Read the model definition and answer for the solid it produces. Units are mm, in the model's axes. Coordinates: 2 decimals unless noted, no trailing zeros. Write each loop counter-clockwise with the first axis right and the second up, starting at its lowest first coordinate (ties: lowest second). Pieces come first, ordered by that corner, then holes. Notation, with made-up numbers: (20, 16.25) -> (56, 16.25) arc R32 ccw to (56, 49.25) -> close; hole circle Ø7 at (28.5, -13). An arc over 180 degrees is marked (long way). Use CSV: the item, a comma, the result in double quotes.
from build123d import *

# Parameters (mm, degrees)
SKETCH1_R           = 100
BOSS_EXTRUDE1_DEPTH = 10
SKETCH2_R           = 15
CUT_EXTRUDE1_DEPTH  = 142.774468788
SKETCH3_R           = 10
CUT_EXTRUDE2_DEPTH  = 7.342697
CIRPATTERN1_START   = 2.65730266
CIRPATTERN1_DEPTH   = 7.34269734


# Read off the part's stored shape, not the designer's step: CirPattern1
with BuildPart() as part:
    # Sketch1 → Boss-Extrude1 (new body)
    with BuildSketch(Plane(origin=(0, 0, 0), x_dir=(1, 0, 0), z_dir=(0, 1, 0))):
        with Locations(Location((0, 0, 0), (0, 0, 270))):
            Circle(SKETCH1_R)
    extrude(amount=BOSS_EXTRUDE1_DEPTH)

    # Sketch2 → Cut-Extrude1 (cut, through all)
    with BuildSketch(Plane(origin=(0, 0, 0), x_dir=(1, 0, 0), z_dir=(0, 1, 0))):
        with Locations(Location((0, 0, 0), (0, 0, 270))):
            Circle(SKETCH2_R)
    extrude(amount=CUT_EXTRUDE1_DEPTH, mode=Mode.SUBTRACT)

    # Sketch3 → Cut-Extrude2 (cut)
    with BuildSketch(Plane(origin=(0, 10, 0), x_dir=(1, 0, 0), z_dir=(0, 1, 0))):
        with Locations((-21.793050468, 0)):
            Circle(SKETCH3_R)
    extrude(amount=-CUT_EXTRUDE2_DEPTH, mode=Mode.SUBTRACT)

    # CirPattern1 outline → CirPattern1 (cut)
    with BuildSketch(Plane(origin=(0, 0, 0), x_dir=(1, 0, 0), z_dir=(0, 1, 0)).offset(CIRPATTERN1_START)):
        with BuildLine():
            ThreePointArc((-13.764411953, -5.961624242), (-18.175613412, -9.322775829), (-23.699395197, -9.816610911))
            ThreePointArc((-23.699395197, -9.816610911), (-22.48108158, -22.48108158), (-9.816610911, -23.699395197))
            ThreePointArc((-9.816610911, -23.699395197), (0, -31.793050468), (9.816610911, -23.699395197))
            ThreePointArc((9.816610911, -23.699395197), (22.48108158, -22.48108158), (23.699395197, -9.816610911))
            ThreePointArc((23.699395197, -9.816610911), (31.793050468, 0), (23.699395197, 9.816610911))
            ThreePointArc((23.699395197, 9.816610911), (22.48108158, 22.48108158), (9.816610911, 23.699395197))
            ThreePointArc((9.816610911, 23.699395197), (0, 31.793050468), (-9.816610911, 23.699395197))
            ThreePointArc((-9.816610911, 23.699395197), (-22.48108158, 22.48108158), (-23.699395197, 9.816610911))
            ThreePointArc((-23.699395197, 9.816610911), (-18.175613412, 9.322775829), (-13.764411953, 5.961624242))
            ThreePointArc((-13.764411953, 5.961624242), (15, 0), (-13.764411953, -5.961624242))
        make_face()
    extrude(amount=CIRPATTERN1_DEPTH, mode=Mode.SUBTRACT)


solid = part.part
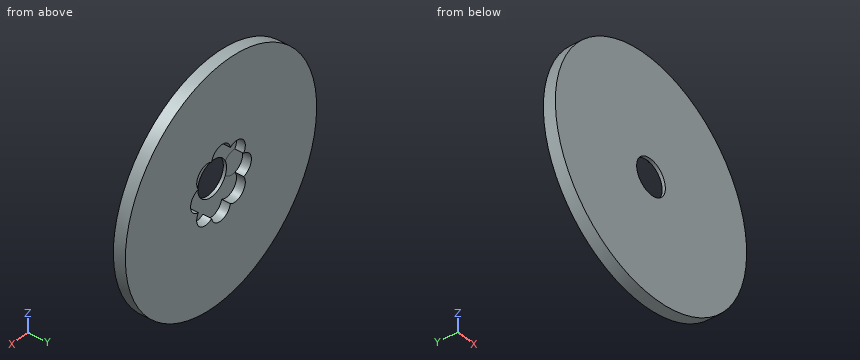
1. A cutting plane is placed at C-C (z = 0). Give the vertices of the cut face in (x, y), and give its area (3 significant figures).
Solutions:
outline,"(-100, 0) -> (-15, 0) -> (-15, 2.66) -> (-31.79, 2.66) -> (-31.79, 10) -> (-100, 10) -> close; (15, 0) -> (100, 0) -> (100, 10) -> (31.79, 10) -> (31.79, 2.66) -> (15, 2.66) -> close"
area,"1,450 mm^2"
2. A cutting plane is placed at D-D (z = -28.5). Give the vertices of the cut face in (x, y).
Solutions:
outline,"(-95.85, 0) -> (95.85, 0) -> (95.85, 10) -> (7.42, 10) -> (7.42, 2.66) -> (-7.42, 2.66) -> (-7.42, 10) -> (-95.85, 10) -> close"
3. Find the intervals of material crossed by line 1 along X through (y, z) = (0.8, 0); line 2 along X through (y, z) = (9, -24); line 3 along X through (y, z) = (5.5, -8.5), in increasing order.
Solutions:
line 1,"x = -100 to -15, 15 to 100"
line 2,"x = -97.08 to -20.53, -10.29 to -9.75, 9.75 to 10.29, 20.53 to 97.08"
line 3,"x = -99.64 to -27.06, 27.06 to 99.64"
4. Each of these flat-tipped pins is pushed along its axis until it touches: pin 1 Ø6 at (x, y) = (-60.5, 2.5) entering from +Z; pin 2 Ø6 at (y, z) = (2, -14) entering from +X; pin 3 Ø3 at (y, z) = (6, -60) entering from +X. Where does it stop, or does it pass through?
Solutions:
pin 1,"stops at z = 81.82"
pin 2,"stops at x = 99.39"
pin 3,"stops at x = 81.1"
5. A cutting plane is placed at B-B (y = 5.75). Give the vertices of the cut face in (x, z).
Solutions:
outline,"circle Ø200 at (0, 0); hole (-23.7, -9.82) arc R10 ccw to (-9.82, -23.7) arc R10 ccw to (9.82, -23.7) arc R10 ccw to (23.7, -9.82) arc R10 ccw to (23.7, 9.82) arc R10 ccw to (9.82, 23.7) arc R10 ccw to (-9.82, 23.7) arc R10 ccw to (-23.7, 9.82) arc R10 ccw to start"
6. A cutting plane is placed at A-A (x = 0). Give the vertices of the cut face in (y, z).
Solutions:
outline,"(0, -100) -> (10, -100) -> (10, -31.79) -> (2.66, -31.79) -> (2.66, -15) -> (0, -15) -> close; (0, 15) -> (2.66, 15) -> (2.66, 31.79) -> (10, 31.79) -> (10, 100) -> (0, 100) -> close"
